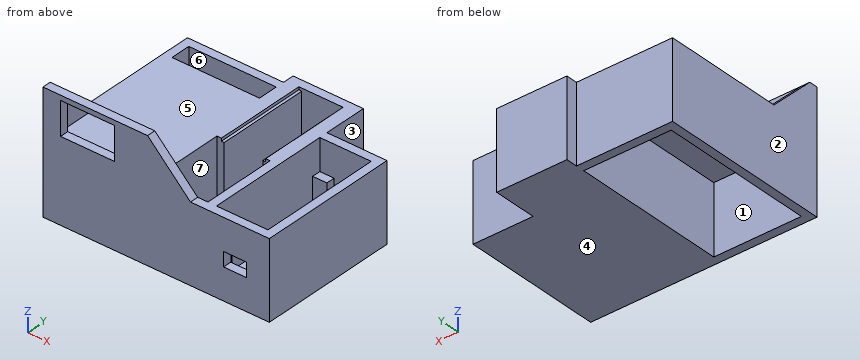
from build123d import *

# Parameters (mm, degrees)
SKETCH1_W            = 1
SKETCH1_H            = 32.4
SKETCH1_W_2          = 13.5
SKETCH1_W_3          = 1.55
SKETCH1_W_4          = 3
SKETCH1_H_2          = 3
SKETCH1_W_5          = 18.6
SKETCH1_H_3          = 26
BOSS_EXTRUDE1_DEPTH  = 3
SKETCH1_5_W          = 3
SKETCH1_5_H          = 3
SKETCH1_5_W_2        = 1
SKETCH1_5_H_2        = 32.4
SKETCH1_5_W_3        = 1.55
BOSS_EXTRUDE2_DEPTH  = 26
BOSS_EXTRUDE4_DEPTH  = 35
SKETCH1_8_W          = 1.55
SKETCH1_8_H          = 32.4
SKETCH1_8_W_2        = 3
SKETCH1_8_H_2        = 3
BOSS_EXTRUDE5_DEPTH  = 27
BOSS_EXTRUDE6_DEPTH  = 3
SKETCH2_3_W          = 3
SKETCH2_3_H          = 3
SKETCH2_3_W_2        = 5
BOSS_EXTRUDE7_DEPTH  = 2
SKETCH2_4_W          = 8
SKETCH2_4_H          = 3
BOSS_EXTRUDE8_DEPTH  = 11
SKETCH2_5_W          = 3
SKETCH2_5_H          = 3
BOSS_EXTRUDE9_DEPTH  = 27
SKETCH5_W            = 30.618778274
SKETCH5_H            = 3
SKETCH5_W_2          = 2.981221726
SKETCH5_H_2          = 60.4
SKETCH5_H_3          = 54.4
BOSS_EXTRUDE11_DEPTH = 3
SKETCH5_5_W          = 30.618778274
SKETCH5_5_H          = 54.4
CUT_EXTRUDE3_DEPTH   = 3
SKETCH5_6_W          = 30.618778274
SKETCH5_6_H          = 3
SKETCH5_6_W_2        = 2.981221726
SKETCH5_6_H_2        = 60.4
BOSS_EXTRUDE12_DEPTH = 27
SKETCH6_W            = 30.618778274
SKETCH6_H            = 47.4
BOSS_EXTRUDE13_DEPTH = 3
SKETCH7_W            = 24.6
SKETCH7_H            = 8
CUT_EXTRUDE4_DEPTH   = 3
SKETCH8_W            = 11
SKETCH8_H            = 3
BOSS_EXTRUDE14_DEPTH = 8
SKETCH2_6_W          = 5
SKETCH2_6_H          = 3
SKETCH2_6_W_2        = 3
BOSS_EXTRUDE15_DEPTH = 16
SKETCH9_W            = 36.6
SKETCH9_H            = 3
BOSS_EXTRUDE16_DEPTH = 15
SKETCH10_W           = 18.8
SKETCH10_H           = 11.60179211
CUT_EXTRUDE5_DEPTH   = 15
BOSS_EXTRUDE17_DEPTH = 3
BOSS_EXTRUDE18_DEPTH = 3


with BuildPart() as part:
    # Sketch1 → Boss-Extrude1 (new body)
    with BuildSketch(Plane.XY):
        with Locations((-16.55, 42.2)):
            Rectangle(SKETCH1_W, SKETCH1_H)
        with Locations((-9.3, 42.2)):
            Rectangle(SKETCH1_W_2, SKETCH1_H)
        with Locations((-2.05, 42.2)):
            Rectangle(SKETCH1_W, SKETCH1_H)
        with Locations((-0.775, 42.2)):
            Rectangle(SKETCH1_W_3, SKETCH1_H)
        with Locations((-17.825, 42.2)):
            Rectangle(SKETCH1_W_3, SKETCH1_H)
        Polygon((-21.6, 0), (-18.6, 0), (-18.6, 26), (-18.6, 58.4), (-21.6, 58.4), align=None)
        with Locations((-20.1, 59.9)):
            Rectangle(SKETCH1_W_4, SKETCH1_H_2)
        Polygon((-1.55, 58.4), (0, 58.4), (0, 61.4), (-18.6, 61.4), (-18.6, 58.4), (-17.05, 58.4), (-16.05, 58.4), (-2.55, 58.4), align=None)
        with Locations((1.5, 59.9)):
            Rectangle(SKETCH1_W_4, SKETCH1_H_2)
        Polygon((0, 26), (0, 0), (3, 0), (3, 58.4), (0, 58.4), align=None)
        with Locations((-9.3, 13)):
            Rectangle(SKETCH1_W_5, SKETCH1_H_3)
        Polygon((-21.6, -3), (-21.6, 0), (-18.6, 0), (0, 0), (3, 0), (3, -3), align=None)
    extrude(amount=BOSS_EXTRUDE1_DEPTH)

    # Sketch1_5 → Boss-Extrude2 (add)
    with BuildSketch(Plane.XY):
        with Locations((-20.1, 59.9)):
            Rectangle(SKETCH1_5_W, SKETCH1_5_H)
        Polygon((-1.55, 58.4), (0, 58.4), (0, 61.4), (-18.6, 61.4), (-18.6, 58.4), (-17.05, 58.4), (-16.05, 58.4), (-2.55, 58.4), align=None)
        with Locations((-2.05, 42.2)):
            Rectangle(SKETCH1_5_W_2, SKETCH1_5_H_2)
        with Locations((-0.775, 42.2)):
            Rectangle(SKETCH1_5_W_3, SKETCH1_5_H_2)
        with Locations((-16.55, 42.2)):
            Rectangle(SKETCH1_5_W_2, SKETCH1_5_H_2)
        with Locations((-17.825, 42.2)):
            Rectangle(SKETCH1_5_W_3, SKETCH1_5_H_2)
        Polygon((-21.6, 0), (-18.6, 0), (-18.6, 26), (-18.6, 58.4), (-21.6, 58.4), align=None)
        with Locations((1.5, 59.9)):
            Rectangle(SKETCH1_5_W, SKETCH1_5_H)
        Polygon((0, 26), (0, 0), (3, 0), (3, 58.4), (0, 58.4), align=None)
        Polygon((-21.6, -3), (-21.6, 0), (-18.6, 0), (0, 0), (3, 0), (3, -3), align=None)
    extrude(amount=BOSS_EXTRUDE2_DEPTH)

    # Sketch1_7 → Boss-Extrude4 (add)
    with BuildSketch(Plane.XY):
        Polygon((-21.6, -3), (-21.6, 0), (-18.6, 0), (0, 0), (3, 0), (3, -3), align=None)
    extrude(amount=BOSS_EXTRUDE4_DEPTH)

    # Sketch1_8 → Boss-Extrude5 (add)
    with BuildSketch(Plane.XY):
        with Locations((-17.825, 42.2)):
            Rectangle(SKETCH1_8_W, SKETCH1_8_H)
        Polygon((-21.6, 0), (-18.6, 0), (-18.6, 26), (-18.6, 58.4), (-21.6, 58.4), align=None)
        with Locations((-20.1, 59.9)):
            Rectangle(SKETCH1_8_W_2, SKETCH1_8_H_2)
        Polygon((-1.55, 58.4), (0, 58.4), (0, 61.4), (-18.6, 61.4), (-18.6, 58.4), (-17.05, 58.4), (-16.05, 58.4), (-2.55, 58.4), align=None)
        with Locations((1.5, 59.9)):
            Rectangle(SKETCH1_8_W_2, SKETCH1_8_H_2)
        Polygon((0, 26), (0, 0), (3, 0), (3, 58.4), (0, 58.4), align=None)
        with Locations((-0.775, 42.2)):
            Rectangle(SKETCH1_8_W, SKETCH1_8_H)
        Polygon((-21.6, -3), (-21.6, 0), (-18.6, 0), (0, 0), (3, 0), (3, -3), align=None)
    extrude(amount=BOSS_EXTRUDE5_DEPTH)

    # Sketch2 → Boss-Extrude6 (add)
    with BuildSketch(Plane(origin=(0, 0, 0), x_dir=(-1, 0, 0), z_dir=(0, 0, -1))):
        Polygon((-8, 0), (-6, 0), (-6, 3), (-3, 3), (-3, 40.2), (-8, 40.2), (-8, 43.2), (-16, 43.2), (-16, 40.2), (-21, 40.2), (-21, 3), (-18, 3), (-18, 0), (-16, 0), align=None)
    extrude(amount=-BOSS_EXTRUDE6_DEPTH)

    # Sketch2_3 → Boss-Extrude7 (add)
    with BuildSketch(Plane(origin=(0, 0, 0), x_dir=(-1, 0, 0), z_dir=(0, 0, -1))):
        with Locations((-4.5, 1.5)):
            Rectangle(SKETCH2_3_W, SKETCH2_3_H)
        Polygon((-3, -3), (-3, 0), (-6, 0), (-8, 0), (-8, -3), align=None)
        with Locations((-19.5, 1.5)):
            Rectangle(SKETCH2_3_W, SKETCH2_3_H)
        Polygon((-21, -3), (-16, -3), (-16, 0), (-18, 0), (-21, 0), align=None)
        with Locations((-22.5, -1.5)):
            Rectangle(SKETCH2_3_W, SKETCH2_3_H)
        Polygon((-8, 43.2), (-3, 43.2), (-3, 46.2), (-24, 46.2), (-24, 43.2), (-24, 0), (-21, 0), (-21, 3), (-21, 40.2), (-21, 43.2), (-16, 43.2), align=None)
        with Locations((-18.5, 41.7)):
            Rectangle(SKETCH2_3_W_2, SKETCH2_3_H)
        with Locations((-5.5, 41.7)):
            Rectangle(SKETCH2_3_W_2, SKETCH2_3_H)
    extrude(amount=-BOSS_EXTRUDE7_DEPTH)

    # Sketch2_4 → Boss-Extrude8 (add)
    with BuildSketch(Plane(origin=(0, 0, 0), x_dir=(-1, 0, 0), z_dir=(0, 0, -1))):
        with Locations((-12, -1.5)):
            Rectangle(SKETCH2_4_W, SKETCH2_4_H)
    extrude(amount=-BOSS_EXTRUDE8_DEPTH)

    # Sketch2_5 → Boss-Extrude9 (add)
    with BuildSketch(Plane(origin=(0, 0, 0), x_dir=(-1, 0, 0), z_dir=(0, 0, -1))):
        Polygon((-3, -3), (-3, 0), (-6, 0), (-8, 0), (-8, -3), align=None)
        Polygon((-21, -3), (-16, -3), (-16, 0), (-18, 0), (-21, 0), align=None)
        with Locations((-22.5, -1.5)):
            Rectangle(SKETCH2_5_W, SKETCH2_5_H)
        Polygon((-8, 43.2), (-3, 43.2), (-3, 46.2), (-24, 46.2), (-24, 43.2), (-24, 0), (-21, 0), (-21, 3), (-21, 40.2), (-21, 43.2), (-16, 43.2), align=None)
    extrude(amount=-BOSS_EXTRUDE9_DEPTH)

    # Sketch5 → Boss-Extrude11 (add)
    with BuildSketch(Plane(origin=(0, 0, 0), x_dir=(-1, 0, 0), z_dir=(0, 0, -1))):
        with Locations((36.909389137, 55.9)):
            Rectangle(SKETCH5_W, SKETCH5_H)
        with Locations((53.709389137, 27.2)):
            Rectangle(SKETCH5_W_2, SKETCH5_H_2)
        with Locations((36.909389137, -1.5)):
            Rectangle(SKETCH5_W, SKETCH5_H)
        with Locations((36.909389137, 27.2)):
            Rectangle(SKETCH5_W, SKETCH5_H_3)
    extrude(amount=-BOSS_EXTRUDE11_DEPTH)

    # Sketch5_5 → Cut-Extrude3 (cut)
    with BuildSketch(Plane(origin=(0, 0, 0), x_dir=(-1, 0, 0), z_dir=(0, 0, -1))):
        with Locations((36.909389137, 27.2)):
            Rectangle(SKETCH5_5_W, SKETCH5_5_H)
    extrude(amount=-CUT_EXTRUDE3_DEPTH, mode=Mode.SUBTRACT)

    # Sketch5_6 → Boss-Extrude12 (add)
    with BuildSketch(Plane(origin=(0, 0, 0), x_dir=(-1, 0, 0), z_dir=(0, 0, -1))):
        with Locations((36.909389137, 55.9)):
            Rectangle(SKETCH5_6_W, SKETCH5_6_H)
        with Locations((53.709389137, 27.2)):
            Rectangle(SKETCH5_6_W_2, SKETCH5_6_H_2)
        with Locations((36.909389137, -1.5)):
            Rectangle(SKETCH5_6_W, SKETCH5_6_H)
    extrude(amount=-BOSS_EXTRUDE12_DEPTH)

    # Sketch6 → Boss-Extrude13 (add)
    with BuildSketch(Plane.XY.offset(27)):
        with Locations((-36.909389137, 23.7)):
            Rectangle(SKETCH6_W, SKETCH6_H)
    extrude(amount=-BOSS_EXTRUDE13_DEPTH)

    # Sketch7 → Cut-Extrude4 (cut)
    with BuildSketch(Plane.XZ.offset(3)):
        with Locations((-9.3, 31)):
            Rectangle(SKETCH7_W, SKETCH7_H)
    extrude(amount=-CUT_EXTRUDE4_DEPTH, mode=Mode.SUBTRACT)

    # Sketch8 → Boss-Extrude14 (add)
    with BuildSketch(Plane(origin=(8, 0, 0), x_dir=(0, 0, -1), z_dir=(1, 0, 0))):
        with Locations((-21.5, -1.5)):
            Rectangle(SKETCH8_W, SKETCH8_H)
    extrude(amount=BOSS_EXTRUDE14_DEPTH)

    # Sketch2_6 → Boss-Extrude15 (add)
    with BuildSketch(Plane(origin=(0, 0, 0), x_dir=(-1, 0, 0), z_dir=(0, 0, -1))):
        with Locations((-5.5, 41.7)):
            Rectangle(SKETCH2_6_W, SKETCH2_6_H)
        with Locations((-18.5, 41.7)):
            Rectangle(SKETCH2_6_W, SKETCH2_6_H)
        with Locations((-19.5, 1.5)):
            Rectangle(SKETCH2_6_W_2, SKETCH2_6_H)
        with Locations((-4.5, 1.5)):
            Rectangle(SKETCH2_6_W_2, SKETCH2_6_H)
    extrude(amount=-BOSS_EXTRUDE15_DEPTH)

    # Sketch9 → Boss-Extrude16 (add)
    with BuildSketch(Plane.XY.offset(27)):
        with Locations((-36.9, -1.5)):
            Rectangle(SKETCH9_W, SKETCH9_H)
    extrude(amount=BOSS_EXTRUDE16_DEPTH)

    # Sketch10 → Cut-Extrude5 (cut)
    with BuildSketch(Plane(origin=(0, -3, 0), x_dir=(-1, 0, 0), z_dir=(0, -1, 0))):
        with Locations((39.656308117, -34.500896055)):
            Rectangle(SKETCH10_W, SKETCH10_H)
    extrude(amount=-CUT_EXTRUDE5_DEPTH, mode=Mode.SUBTRACT)

    # Sketch11 → Boss-Extrude17 (add)
    with BuildSketch(Plane(origin=(0, -3, 0), x_dir=(-1, 0, 0), z_dir=(0, -1, 0))):
        Polygon((18.6, -42), (18.6, -27), (3.6, -27), align=None)
    extrude(amount=-BOSS_EXTRUDE17_DEPTH)

    # Sketch12 → Boss-Extrude18 (add)
    with BuildSketch(Plane.ZY.offset(55.2)):
        Polygon((27, 0), (42, 0), (27, 15), align=None)
    extrude(amount=-BOSS_EXTRUDE18_DEPTH)


solid = part.part
Work out the finished part from the listing and answer in its coordinate system (mm). Face numbers are marked on the shaded views. A direction names the side the tool comes from. Give positions to 0.01 mm unless a question says otherwise; leave off trailing zeros. Write each loop counter-clockwise with the first axis right and the second up, starting at its lowest first coordinate (ties: lowest second). Pieces come first, ordered by that corner, then holes. Notation, with made-up numbers: M 38,23 L 54,23 A25 ccw 54,56 Z; hole C -24,-13.75 d1. An arc over 180 degrees is marked long. Answer as CSV lines item,"result".
Q1. A cutting plane is placed at D-D on z = 32.5. Write down the section's boundary in (x, y).
A:
outline,"M -55.2,-3 L -49.06,-3 L -49.06,0 L -52.2,0 L -52.2,9.5 L -55.2,9.5 Z; M -30.26,-3 L -9.1,-3 L -9.1,0 L -30.26,0 Z"
Q2. A tool of negligible diameter and unlimited length cuts with its end or side. For the marked faces 5, 6 and 7, from which of +Z, -Z, +X, -X, +Y, -Y can it reach the whole face along a straight path? Write none if from no direction.
A:
face 5,"+Z, +X, +Y"
face 6,"+Z, -Z"
face 7,"+Z"
Q3. The mould has two halves that part along X. Classify the marked faces 1, 2, 3 and 4: +X half, -X half, draft (parallel to the pull), parting line (faces both ways), or undercut.
A:
face 1,"undercut"
face 2,"-X half"
face 3,"+X half"
face 4,"draft"
Q4. A cutting plane is placed at C-C on y = 56. Write down the section's boundary in (x, z).
A:
outline,"M -55.2,0 L 3,0 L 3,27 L -1.55,27 L -1.55,26 L -2.55,26 L -2.55,3 L -16.05,3 L -16.05,26 L -17.05,26 L -17.05,27 L -55.2,27 Z"
Q5. A cutting plane is placed at A-A on x = -26. Write down the section's boundary in (y, z), plus the area to 3 significant figures.
A:
outline,"M -3,0 L 0,0 L 0,24 L 47.4,24 L 47.4,27 L 0,27 L 0,42 L -3,42 Z; M 54.4,0 L 57.4,0 L 57.4,27 L 54.4,27 Z"
area,"349 mm²"
Q6. A cutting plane is placed at B-B on z = 10. Count the separate pieces of the cut face and the enclosed holes in it, plus the area to 3 significant figures.
A:
separate pieces,"1"
enclosed holes,"3"
area,"1,330 mm²"
Q7. Given P1, Ø2.5, axis at x = -35, z = 25.5, coming from the +Y side; P2, Ø2, axis at x = -23.5, y = 22.5, coming from the -Z side; P3, Ø2, axis at y = 60, z = 19.5, coming from the -X side, each flat-ended and moving along its own axis, determine where each tip first touches the part or whether it passes through.
A:
P1,"stops at y = 57.4"
P2,"stops at z = 24"
P3,"stops at x = -21.6"
Q8. Find the intervals of material crossed by probe 1 along X at (y, z) = (8, 8); probe 2 along X at (y, z) = (35, 10.5); probe 3 along X at (y, z) = (37.5, 25.5), in increasing order. Write a range as [from, to].
A:
probe 1,"x = [-55.2, -52.22], [-21.6, -18.6], [0, 3], [21, 24]"
probe 2,"x = [-55.2, -52.22], [-21.6, -16.05], [-2.55, 3], [21, 24]"
probe 3,"x = [-55.2, -16.05], [-2.55, 3], [21, 24]"
